from build123d import *

# Parameters (mm, degrees)
SKETCH1_R           = 22
BOSS_EXTRUDE1_DEPTH = 10
CUT_EXTRUDE2_DEPTH  = 5.5
SKETCH15_W          = 18
SKETCH15_H          = 24.118038922
CUT_EXTRUDE3_DEPTH  = 3
SKETCH16_R          = 4
BOSS_EXTRUDE2_DEPTH = 10
CUT_EXTRUDE4_START  = 20
SKETCH8_W           = 1.2
SKETCH8_H           = 10
CUT_EXTRUDE4_DEPTH  = 5
SKETCH17_W          = 4
SKETCH17_H          = 1.75
BOSS_EXTRUDE3_DEPTH = 1
SKETCH18_W          = 4.25
SKETCH18_H          = 1.737607108
BOSS_EXTRUDE4_DEPTH = 1
SKETCH22_R          = 1.5
CUT_EXTRUDE7_DEPTH  = 7


with BuildPart() as part:
    # Sketch1 → Boss-Extrude1 (new body)
    with BuildSketch(Plane(origin=(0, 0, 0), x_dir=(0, 0, -1), z_dir=(1, 0, 0))):
        Circle(SKETCH1_R)
    extrude(amount=BOSS_EXTRUDE1_DEPTH)

    # Sketch13 → Cut-Extrude2 (cut)
    with BuildSketch(Plane(origin=(0, 0, 0), x_dir=(0, 0, -1), z_dir=(1, 0, 0))):
        with BuildLine():
            Line((-2.670420152, -16.85816067), (-2.670420152, -16.530371213))
            Line((-2.670420152, -16.530371213), (-4.762392892, -10))
            Line((-4.762392892, -10), (-4.762392892, -6.943148259))
            Line((-4.762392892, -6.943148259), (-6.5, -6.943148259))
            Line((-6.5, -6.943148259), (-6.5, 19.556851741))
            Line((-6.5, 19.556851741), (6.5, 19.556851741))
            Line((6.5, 19.556851741), (6.5, -6.943148259))
            Line((6.5, -6.943148259), (4.762392892, -6.943148259))
            Line((4.762392892, -6.943148259), (4.762392892, -10))
            Line((4.762392892, -10), (2.670420152, -16.530371213))
            Line((2.670420152, -16.530371213), (2.670420152, -16.85816067))
            Line((2.670420152, -16.85816067), (2.670420152, -21.837327131))
            ThreePointArc((2.670420152, -21.837327131), (1.836835043, -21.92318492), (1.000584871, -21.977234355))
            Line((1.000584871, -21.977234355), (0, -25.25))
            Line((0, -25.25), (-1.000584871, -21.977234355))
            ThreePointArc((-1.000584871, -21.977234355), (-1.836835043, -21.92318492), (-2.670420152, -21.837327131))
            Line((-2.670420152, -21.837327131), (-2.670420152, -16.85816067))
        make_face()
    extrude(amount=CUT_EXTRUDE2_DEPTH, mode=Mode.SUBTRACT)

    # Sketch15 → Cut-Extrude3 (cut)
    with BuildSketch(Plane.ZY):
        with Locations((0, 5.115871202)):
            Rectangle(SKETCH15_W, SKETCH15_H)
    extrude(amount=-CUT_EXTRUDE3_DEPTH, mode=Mode.SUBTRACT)

    # Sketch16 → Boss-Extrude2 (add)
    with BuildSketch(Plane(origin=(10, 0, 0), x_dir=(0, 0, -1), z_dir=(1, 0, 0))):
        Circle(SKETCH16_R)
    extrude(amount=BOSS_EXTRUDE2_DEPTH)

    # Sketch8 → Cut-Extrude4 (cut)
    with BuildSketch(Plane(origin=(0, 0, 0), x_dir=(0, 0, -1), z_dir=(1, 0, 0)).offset(CUT_EXTRUDE4_START)):
        Rectangle(SKETCH8_W, SKETCH8_H)
    extrude(amount=-CUT_EXTRUDE4_DEPTH, mode=Mode.SUBTRACT)

    # Sketch17 → Boss-Extrude3 (add)
    with BuildSketch(Plane(origin=(0, -6.943148259, 0), x_dir=(1, 0, 0), z_dir=(0, 1, 0))):
        with Locations((2, 5.637392892)):
            Rectangle(SKETCH17_W, SKETCH17_H)
    extrude(amount=BOSS_EXTRUDE3_DEPTH)

    # Sketch18 → Boss-Extrude4 (add)
    with BuildSketch(Plane(origin=(0, -6.943148259, 0), x_dir=(1, 0, 0), z_dir=(0, 1, 0))):
        with Locations((2.125, -5.631196446)):
            Rectangle(SKETCH18_W, SKETCH18_H)
    extrude(amount=BOSS_EXTRUDE4_DEPTH)

    # Sketch22 → Cut-Extrude7 (cut)
    with BuildSketch(Plane(origin=(0, 0, 0), x_dir=(0, 0, -1), z_dir=(1, 0, 0))):
        with Locations((-14, 0)):
            Circle(SKETCH22_R)
        with Locations((14, 0)):
            Circle(SKETCH22_R)
    extrude(amount=CUT_EXTRUDE7_DEPTH, mode=Mode.SUBTRACT)


solid = part.part
Source: CAD feature listing. Evaluate the final solid. Frame: model axes, mm. A direction names the side the tool comes from. Coordinates: 2 decimals unless noted, no trailing zeros. Loops run counter-clockwise (first coordinate to the right, second up) from the corner with the lowest first, then second, coordinate; pieces in that order, holes last. Notation, with made-up numbers: (73.5, -31) - (88.5, -31) arc R11 ccw to (88.5, -13) - close; hole circle Ø6 at (-6.5, 52.5). An arc over 180 degrees is marked (long way). One line per item, written item: value. Start each with the question number.
1. Section C-C (y = 19). Return the cut outline in (x, z).
2. Mould query, pull axis Z, two halves, no side actions, for faces 4 (the flat face through (15, 0, 0)), 5 (the flat face through (0, -0.2, -9.5)), 6 (the cylindrical face through (4.93, -21.477, 4.769)). Classes: pulls with the +Z half, pulls with the -Z half, needs draft (parallel to the pull), parting line crosses it, or undercut.
3. Set-up query: faces 1 (the flat face through (5, -6.943, -6)), 2 (the flat face through (7, 0, 14)), 3 (the flat face through (18, 0, -0.6)). Return all of +Z, -Z, +X, -X, +Y, -Y with unobstructed straight access to the full face (end or side cutting, diameter ignored); none if empty.
4. Section B-B (x = 15.75). Return the cut outline in (y, z), and give its area (3 significant figures).
5. Contact query for flat-ended pins moving along their axis: P1, Ø6, axis at x = 11.5, y = -14.5, coming from the +Z side; P2, Ø0.8, axis at y = -6.5, z = -5.5, coming from the +X side; P3, Ø2, axis at x = 1, z = 7.5, coming from the -Y side; P4, Ø5, axis at y = -7, z = -16.5, coming from the -X side. Output: stop coordinate, or through.
6. Section D-D (x = 10.75). Return the cut outline in (y, z).
7. Section A-A (z = 0). Return the cut outline in (x, y).
8. Ray query, L1, parallel to X at y = -11.5, z = -15.5; L2, parallel to Y at x = 4.75, z = 14; L3, parallel to Z at x = 1, y = 3. Return the intervals inside material, ascending.
Verdict:
1. outline: (0, -11.09) - (10, -11.09) - (10, 11.09) - (0, 11.09) - (0, 6.5) - (5.5, 6.5) - (5.5, -6.5) - (0, -6.5) - close
2. face 4: undercut
2. face 5: needs draft
2. face 6: parting line crosses it
3. face 1: none
3. face 2: -X
3. face 3: +X, +Y, -Y
4. outline: (-3.95, -0.6) arc R4 ccw to (3.95, -0.6) - close; (-3.95, 0.6) - (3.95, 0.6) arc R4 ccw to start
4. area: 40.7 mm2
5. P1: stops at z = 18.5
5. P2: stops at x = 10
5. P3: stops at y = -21.02
5. P4: stops at x = 0
6. outline: circle Ø8 at (0, 0)
7. outline: (0, 19.56) - (5.5, 19.56) - (5.5, -22) - (10, -22) - (10, -4) - (15, -4) - (15, 4) - (10, 4) - (10, 22) - (0, 22) - close
8. L1: x = 0 to 10
8. L2: y = -16.97 to -1.5, 1.5 to 16.97
8. L3: z = -21.79 to -9, 9 to 21.79
